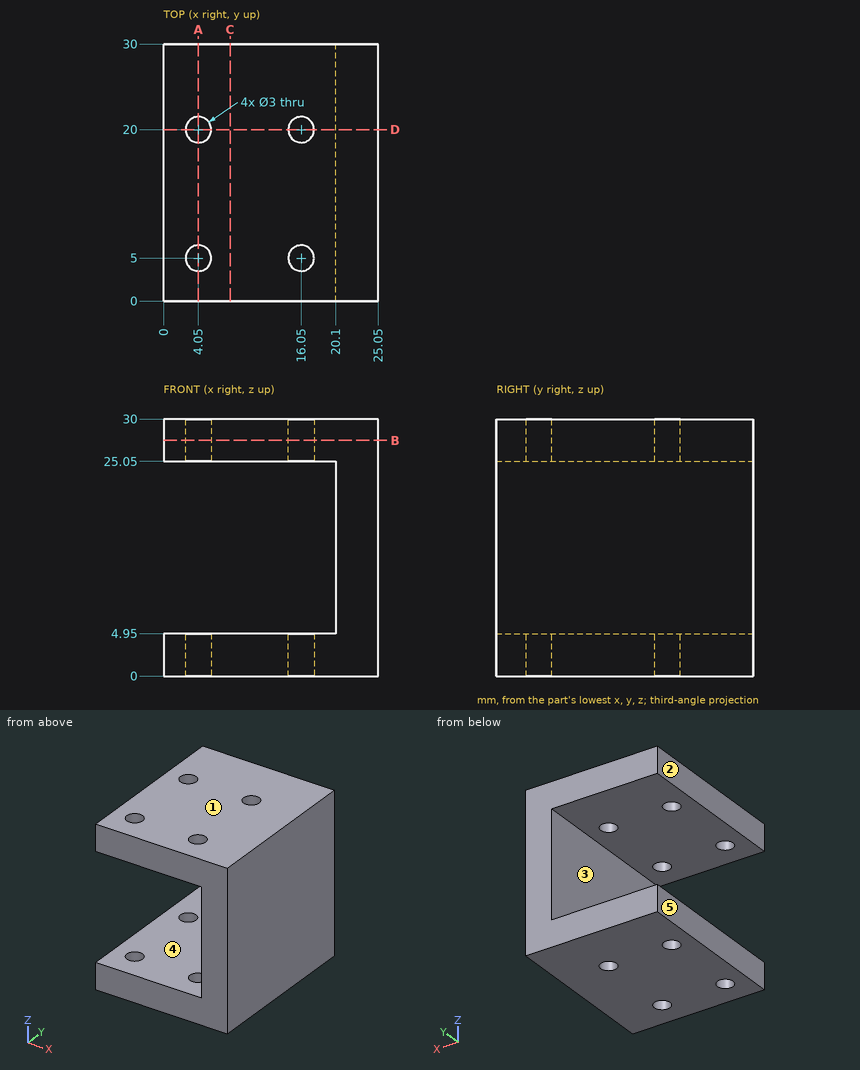
Print and shaded views of the part. All mm, measured from the part's lowest x, y and z. A direction names the side the tool comes from. Coordinates: 2 decimals unless noted, no trailing zeros. Loops run counter-clockwise (first coordinate to the right, second up) from the corner with the lowest first, then second, coordinate; pieces in that order, holes last. Notation, with made-up numbers: (54.5, 83) -> (76.5, 83) arc R23 cw to (76.5, 100) -> close; hole circle Ø2 at (21, 86.5). An arc over 180 degrees is marked (long way). Use a Markdown table: item, result. Add a question column.
Item 1: Which spindle directions (+Z, -Z, +X, -X, +Y, -Y) get a long thin tool onto all of the face, cutting with end or side? Do the marked faces 4 and 5. Say none if no direction does.
Item 2: Band-saw the part on A-A on x = 4.05. Write the cut outline in (y, z), plus the area to 3 significant figures.
Item 3: Pull direction Z, two halves, no side cores. Call the marked faces 1, 2 and 3: +Z half, -Z half, draft (parallel to the pull), parting line (faces both ways), or undercut.
Item 4: Probe probe 1 along Y at (x, z) = (4.05, 26.8); probe 2 along X at (y, z) = (20, 2.7); probe 3 along Z at (x, y) = (3.5, 7.25). List the from-to ranges inside material, lowest first.
Item 5: Band-saw the part on C-C on x = 7.75. Write the cut outline in (y, z), plus the area to 3 significant figures.
Item 6: Band-saw the part on B-B on z = 27.5. Write the cut outline in (x, y), plus the area to 3 significant figures.
Item 7: Band-saw the part on D-D on y = 20. Write the cut outline in (x, z), plus the area to 3 significant figures.
Geometry says:
| question | item | result |
|---|---|---|
| 1 | face 4 | -X, +Y, -Y |
| 1 | face 5 | +Z, -Z, -X, +Y, -Y |
| 2 | outline | (0, 0) -> (3.5, 0) -> (3.5, 4.95) -> (0, 4.95) -> close; (0, 25.05) -> (3.5, 25.05) -> (3.5, 30) -> (0, 30) -> close; (6.5, 0) -> (18.5, 0) -> (18.5, 4.95) -> (6.5, 4.95) -> close; (6.5, 25.05) -> (18.5, 25.05) -> (18.5, 30) -> (6.5, 30) -> close; (21.5, 0) -> (30, 0) -> (30, 4.95) -> (21.5, 4.95) -> close; (21.5, 25.05) -> (30, 25.05) -> (30, 30) -> (21.5, 30) -> close |
| 2 | area | 238 mm² |
| 3 | face 1 | +Z half |
| 3 | face 2 | draft |
| 3 | face 3 | undercut |
| 4 | probe 1 | 0 to 3.5, 6.5 to 18.5, 21.5 to 30 |
| 4 | probe 2 | 0 to 2.55, 5.55 to 14.55, 17.55 to 25.05 |
| 4 | probe 3 | 0 to 4.95, 25.05 to 30 |
| 5 | outline | (0, 0) -> (30, 0) -> (30, 4.95) -> (0, 4.95) -> close; (0, 25.05) -> (30, 25.05) -> (30, 30) -> (0, 30) -> close |
| 5 | area | 297 mm² |
| 6 | outline | (0, 0) -> (25.05, 0) -> (25.05, 30) -> (0, 30) -> close; hole circle Ø3 at (4.05, 5); hole circle Ø3 at (4.05, 20); hole circle Ø3 at (16.05, 5); hole circle Ø3 at (16.05, 20) |
| 6 | area | 723 mm² |
| 7 | outline | (0, 0) -> (2.55, 0) -> (2.55, 4.95) -> (0, 4.95) -> close; (0, 25.05) -> (2.55, 25.05) -> (2.55, 30) -> (0, 30) -> close; (5.55, 0) -> (14.55, 0) -> (14.55, 4.95) -> (5.55, 4.95) -> close; (5.55, 25.05) -> (14.55, 25.05) -> (14.55, 30) -> (5.55, 30) -> close; (17.55, 0) -> (25.05, 0) -> (25.05, 30) -> (17.55, 30) -> (17.55, 25.05) -> (20.1, 25.05) -> (20.1, 4.95) -> (17.55, 4.95) -> close |
| 7 | area | 288 mm² |
